from build123d import *

# Parameters (mm, degrees)
F2_DEPTH = 31.75
F3_DEPTH = 12.7
F1_R     = 15
F4_DEPTH = 9.525
F1_R_2   = 3
F5_DEPTH = 3.175
F6_W     = 6
F6_H     = 13.05


with BuildPart() as f2:
    # F1 (on Top) → F2 (new body)
    with BuildSketch(Plane.XY):
        with BuildLine():
            ThreePointArc((-32, 31), (-44.5533388199, 0), (-32, -31))
            Line((-32, -31), (-32, 31))
        make_face()
    extrude(amount=F2_DEPTH)



with BuildPart() as f2b:
    # F1 (on Top) → F2, piece 2 (new body)
    with BuildSketch(Plane.XY):
        with BuildLine():
            Line((32, 31), (32, -31))
            ThreePointArc((32, -31), (44.5533388199, 0), (32, 31))
        make_face()
    extrude(amount=F2_DEPTH)


with BuildPart() as f3:
    # F1 (on Top) → F3 (new body)
    with BuildSketch(Plane.XY):
        with BuildLine():
            ThreePointArc((40.4111525448, -40.4111525448), (52.799715283, -21.8703581597), (57.15, 0))
            ThreePointArc((57.15, 0), (-21.8703581597, 52.799715283), (-40.4111525448, -40.4111525448))
            Line((-40.4111525448, -40.4111525448), (-32, -31))
            ThreePointArc((-32, -31), (-44.5533388199, 0), (-32, 31))
            ThreePointArc((-32, 31), (0, 44.5533388199), (32, 31))
            ThreePointArc((32, 31), (44.5533388199, 0), (32, -31))
            Line((32, -31), (40.4111525448, -40.4111525448))
        make_face()
        with BuildLine():
            ThreePointArc((32, 31), (0, 44.5533388199), (-32, 31))
            Line((-32, 31), (32, 31))
        make_face()
    extrude(amount=F3_DEPTH)


with BuildPart() as f4:
    # F1 (on Top) → F4 (new body)
    with BuildSketch(Plane.XY):
        Circle(F1_R)
    extrude(amount=F4_DEPTH)


with BuildPart() as f4b:
    # F1 (on Top) → F4, piece 2 (new body)
    with BuildSketch(Plane.XY):
        with Locations((16, -31)):
            Circle(F1_R_2)
    extrude(amount=F4_DEPTH)


with BuildPart() as f4c:
    # F1 (on Top) → F4, piece 3 (new body)
    with BuildSketch(Plane.XY):
        with Locations((-16, -31)):
            Circle(F1_R_2)
    extrude(amount=F4_DEPTH)


with BuildPart() as f2_1:
    add(f2.part)

    add(f2b.part)  # F5 merges F2b

    add(f3.part)  # F5 merges F3

    add(f4.part)  # F5 merges F4

    add(f4b.part)  # F5 merges F4b

    add(f4c.part)  # F5 merges F4c
    # F1 (on Top) → F5 (join)
    with BuildSketch(Plane.XY):
        with BuildLine():
            Line((-32, -31), (-40.4111525448, -40.4111525448))
            ThreePointArc((-40.4111525448, -40.4111525448), (0, -57.15), (40.4111525448, -40.4111525448))
            Line((40.4111525448, -40.4111525448), (32, -31))
            Line((32, -31), (32, 31))
            Line((32, 31), (-32, 31))
            Line((-32, 31), (-32, -31))
        make_face()
        with Locations((-16, -31)):
            Circle(F1_R_2, mode=Mode.SUBTRACT)
        with Locations((16, -31)):
            Circle(F1_R_2, mode=Mode.SUBTRACT)
        Circle(F1_R, mode=Mode.SUBTRACT)
        with BuildLine():
            ThreePointArc((40.4111525448, -40.4111525448), (52.799715283, -21.8703581597), (57.15, 0))
            ThreePointArc((57.15, 0), (-21.8703581597, 52.799715283), (-40.4111525448, -40.4111525448))
            Line((-40.4111525448, -40.4111525448), (-32, -31))
            ThreePointArc((-32, -31), (-44.5533388199, 0), (-32, 31))
            ThreePointArc((-32, 31), (0, 44.5533388199), (32, 31))
            ThreePointArc((32, 31), (44.5533388199, 0), (32, -31))
            Line((32, -31), (40.4111525448, -40.4111525448))
        make_face()
        with BuildLine():
            Line((32, 31), (32, -31))
            ThreePointArc((32, -31), (44.5533388199, 0), (32, 31))
        make_face()
        with BuildLine():
            ThreePointArc((32, 31), (0, 44.5533388199), (-32, 31))
            Line((-32, 31), (32, 31))
        make_face()
        with BuildLine():
            ThreePointArc((-32, 31), (-44.5533388199, 0), (-32, -31))
            Line((-32, -31), (-32, 31))
        make_face()
        with Locations((-16, -31)):
            Circle(F1_R_2)
        with Locations((16, -31)):
            Circle(F1_R_2)
        Circle(F1_R)
    extrude(amount=-F5_DEPTH)

    # F6 (on face) → F7 (revolve, cut)
    with BuildSketch(Plane.YZ.offset(-32)):
        with Locations((-28, 19.225)):
            Rectangle(F6_W, F6_H)
    revolve(axis=Axis((0, 0, 0), (0, 0, -1)), mode=Mode.SUBTRACT)


solid = f2_1.part
Geometry: final body of the model. Coordinates: model frame, mm. A direction names the side the tool comes from. Give positions to 0.01 mm unless a question says otherwise; leave off trailing zeros. Write each loop counter-clockwise with the first axis right and the second up, starting at its lowest first coordinate (ties: lowest second). Pieces come first, ordered by that corner, then holes. Notation, with made-up numbers: (-33.5, -32) - (24.5, -32) arc R9 cw to (24.5, -27) - close; hole circle Ø3 at (-25, -18). An arc over 180 degrees is marked (long way). Return JSON: item names as keys, results as strings. Group by question number.
1) Line query: line 1 (Z direction, x = -5, y = 8) (3 decimals); line 2 (Z direction, x = -22.5, y = -26) (3 decimals); line 3 (X direction, y = -8, z = 17.5). Output: solid intervals per line, ascending.
2) Set-up query: faces 1 (the flat face through (0, 31, 6)), 2 (the cylindrical face through (-40.606, -0.377, 19.316)), 3 (the flat face through (0, 0, 9.525)). Return all of +Z, -Z, +X, -X, +Y, -Y with unobstructed straight access to the full face (end or side cutting, diameter ignored); none if empty.
3) First-contact query: P1, Ø1.5, axis at y = -26, z = 8.5, coming from the +X side; P2, Ø5, axis at x = 15.5, y = -29.5, coming from the +Z side (3 decimals); P3, Ø8, axis at x = -19.5, y = -5.5, coming from the +Z side. Flat tips, straight axial feed; report the tip coordinate or a pass-through.
4) Section D-D on x = 2. Return the cut outline in (y, z) (3 decimals), plus the area to 3 significant figures.
5) Section C-C on x = -37.5. Return the cut outline in (y, z) (3 decimals), plus the area to 3 significant figures.
6) Section B-B on z = 24. Return the cut outline in (x, y).
7) Mould query, pull axis X, two halves, no side actions, for faces 4 (the flat face through (41, 0, 25.75)), 5 (the cylindrical face through (44.55, -0.48, 28.71)), 6 (the cylindrical face through (-19, -31, 5)), 7 (the cylindrical face through (-2.473, 57.096, 4.874)). Classes: released by +X, released by -X, zero draft, split by the parting line, or undercut.
8) Section A-A on y = 0. Return the cut outline in (x, z) (3 decimals), plus the area to 3 significant figures.
Filled in:
{
 "1": {"line 1": "z = -3.175 to 9.525", "line 2": "z = -3.175 to 0", "line 3": "x = -39.81 to -32, 32 to 39.81"},
 "2": {"face 1": "+Z", "face 2": "-X", "face 3": "+Z, -Y"},
 "3": {"P1": "stops at x = 51.27", "P2": "stops at z = 9.525", "P3": "stops at z = 0"},
 "4": {"outline": "(-57.115, -3.175) - (57.115, -3.175) - (57.115, 12.7) - (31, 12.7) - (31, 0) - (14.866, 0) - (14.866, 9.525) - (-14.866, 9.525) - (-14.866, 0) - (-57.115, 0) - close", "area": "978 mm^2"},
 "5": {"outline": "(-43.126, -3.175) - (43.126, -3.175) - (43.126, 12.7) - (15.58, 12.7) - (15.58, 25.75) - (24.057, 25.75) - (24.057, 31.75) - (-24.057, 31.75) - (-24.057, 25.75) - (-15.58, 25.75) - (-15.58, 12.7) - (-37.154, 12.7) - (-37.154, 0) - (-43.126, 0) - close", "area": "1,990 mm^2"},
 "6": {"outline": "(-32, -25) - (-32, 25) arc R40.61 ccw to start; (32, -25) arc R40.61 ccw to (32, 25) - close"},
 "7": {"face 4": "zero draft", "face 5": "released by +X", "face 6": "undercut", "face 7": "split by the parting line"},
 "8": {"outline": "(-57.15, -3.175) - (57.15, -3.175) - (57.15, 12.7) - (40.608, 12.7) - (40.608, 25.75) - (44.553, 25.75) - (44.553, 31.75) - (32, 31.75) - (32, 0) - (15, 0) - (15, 9.525) - (-15, 9.525) - (-15, 0) - (-32, 0) - (-32, 31.75) - (-44.553, 31.75) - (-44.553, 25.75) - (-40.608, 25.75) - (-40.608, 12.7) - (-57.15, 12.7) - close", "area": "1,660 mm^2"}
}
